For this review, take the finished solid that the model builds, in its own axes (mm). A direction names the side the tool comes from. Round coordinates to 2 decimals unless told otherwise and drop trailing zeros. Order: outer loops, then holes, each group sorted by start corner. A loop starts at its lowest first (then second) coordinate and runs counter-clockwise, first axis right, second up. Notation, with made-up numbers: (80.5, 82) - (103.5, 82) arc R27 ccw to (103.5, 109) - close; hole circle Ø7 at (72.5, 80.25). An arc over 180 degrees is marked (long way). One line per question, with ' | ' between items.
```python
from build123d import *

# Parameters (mm, degrees)
SKETCH1_R           = 23
SKETCH1_R_2         = 21
BOSS_EXTRUDE1_DEPTH = 20
CUT_EXTRUDE1_START  = 19.798989767
CUT_EXTRUDE1_DEPTH  = 3.113888708
BOSS_EXTRUDE2_START = -1
SKETCH3_R           = 21
SKETCH3_R_2         = 6
BOSS_EXTRUDE2_DEPTH = 1
BOSS_EXTRUDE3_START = 8
SKETCH4_R           = 6
BOSS_EXTRUDE3_DEPTH = 8


# Read off the part's stored shape, not the designer's step: Cut-Extrude1
with BuildPart() as part:
    # Sketch1 → Boss-Extrude1 (new body)
    with BuildSketch(Plane(origin=(0, 0, 0), x_dir=(0, 0, -1), z_dir=(1, 0, 0))):
        Circle(SKETCH1_R)
        Circle(SKETCH1_R_2, mode=Mode.SUBTRACT)
    extrude(amount=BOSS_EXTRUDE1_DEPTH)

    # Cut-Extrude1 outline → Cut-Extrude1 (cut)
    with BuildSketch(Plane(origin=(0, 0, 0), x_dir=(1, 0, 0), z_dir=(0, 1, 0)).offset(CUT_EXTRUDE1_START)):
        with BuildLine():
            add(Edge.make_bspline(
                [(7.15, 7), (7.818022917, 7), (8.466048034, 6.72160004), (9.377693338, 5.805707302), (9.644739555, 5.166655745), (9.655100007, 3.873398622), (9.398895769, 3.221423625), (8.466344312, 2.273000364), (7.817770221, 2), (7.15, 2)],
                knots=[0, 0, 0, 0, 0.25, 0.25, 0.5, 0.5, 0.75, 0.75, 1, 1, 1, 1], degree=3))
            Line((7.15, 7), (3.85, 7))
            add(Edge.make_bspline(
                [(3.85, 7), (3.181977083, 7), (2.533951966, 6.72160004), (1.622306662, 5.805707302), (1.355260445, 5.166655745), (1.344899993, 3.873398622), (1.601104231, 3.221423625), (2.533655688, 2.273000364), (3.182229779, 2), (3.85, 2)],
                knots=[0, 0, 0, 0, 0.25, 0.25, 0.5, 0.5, 0.75, 0.75, 1, 1, 1, 1], degree=3))
            Line((3.85, 2), (7.15, 2))
        make_face()
        with BuildLine():
            Line((3.85, -7), (7.15, -7))
            add(Edge.make_bspline(
                [(7.15, -7), (7.818022917, -7), (8.466048034, -6.72160004), (9.377693338, -5.805707302), (9.644739555, -5.166655745), (9.655100007, -3.873398622), (9.398895769, -3.221423625), (8.466344312, -2.273000364), (7.817770221, -2), (7.15, -2)],
                knots=[0, 0, 0, 0, 0.25, 0.25, 0.5, 0.5, 0.75, 0.75, 1, 1, 1, 1], degree=3))
            Line((7.15, -2), (3.85, -2))
            add(Edge.make_bspline(
                [(3.85, -7), (3.181977083, -7), (2.533951966, -6.72160004), (1.622306662, -5.805707302), (1.355260445, -5.166655745), (1.344899993, -3.873398622), (1.601104231, -3.221423625), (2.533655688, -2.273000364), (3.182229779, -2), (3.85, -2)],
                knots=[0, 0, 0, 0, 0.25, 0.25, 0.5, 0.5, 0.75, 0.75, 1, 1, 1, 1], degree=3))
        make_face()
    extrude(amount=CUT_EXTRUDE1_DEPTH, mode=Mode.SUBTRACT)

    # Sketch3 → Boss-Extrude2 (add)
    with BuildSketch(Plane(origin=(20, 0, 0), x_dir=(0, 0, -1), z_dir=(1, 0, 0)).offset(BOSS_EXTRUDE2_START)):
        Circle(SKETCH3_R)
        Circle(SKETCH3_R_2, mode=Mode.SUBTRACT)
    extrude(amount=BOSS_EXTRUDE2_DEPTH)

    # Sketch4 → Boss-Extrude3 (add)
    with BuildSketch(Plane.ZY.offset(-19).offset(BOSS_EXTRUDE3_START)):
        with BuildLine():
            Line((7.937253933, -1), (20.976176963, -1))
            ThreePointArc((20.976176963, -1), (21, 0), (20.976176963, 1))
            Line((20.976176963, 1), (7.937253933, 1))
            ThreePointArc((7.937253933, 1), (5.656854249, 5.656854249), (1, 7.937253933))
            Line((1, 7.937253933), (1, 20.976176963))
            ThreePointArc((1, 20.976176963), (0, 21), (-1, 20.976176963))
            Line((-1, 20.976176963), (-1, 7.937253933))
            ThreePointArc((-1, 7.937253933), (-5.656854249, 5.656854249), (-7.937253933, 1))
            Line((-7.937253933, 1), (-20.976176963, 1))
            ThreePointArc((-20.976176963, 1), (-21, 0), (-20.976176963, -1))
            Line((-20.976176963, -1), (-7.937253933, -1))
            ThreePointArc((-7.937253933, -1), (-5.656854249, -5.656854249), (-1, -7.937253933))
            Line((-1, -7.937253933), (-1, -20.976176963))
            ThreePointArc((-1, -20.976176963), (0, -21), (1, -20.976176963))
            Line((1, -20.976176963), (1, -7.937253933))
            ThreePointArc((1, -7.937253933), (5.656854249, -5.656854249), (7.937253933, -1))
        make_face()
        with Locations(Location((0, 0, 0), (0, 0, 180))):
            Circle(SKETCH4_R, mode=Mode.SUBTRACT)
    extrude(amount=-BOSS_EXTRUDE3_DEPTH)


solid = part.part
```
(1) Insertion check: pin 1 (3 mm diameter, centred on x = 10, y = 8, fed in from +Z); pin 2 (2.5 mm diameter, centred on x = 13.5, z = 15.5, fed in from +Y); pin 3 (10 mm diameter, centred on x = 7, y = -16, fed in from +Z). Each pin has a flat end and moves straight along its axis. Give the tip position at first contact, or say it passes through.
Output values:
pin 1: z = 22.06 | pin 2: y = 18.05 | pin 3: z = 20.2
(2) We need section D-D on x = 13.5. State the section outline as (y, z) points, plus the area to 3 significant figures.
Output values:
outline: circle Ø46 at (0, 0); hole (-20.98, -1) arc R21 ccw to (-1, -20.98) - (-1, -7.94) arc R8 cw to (-7.94, -1) - close; hole (-20.98, 1) - (-7.94, 1) arc R8 cw to (-1, 7.94) - (-1, 20.98) arc R21 ccw to start; hole circle Ø12 at (0, 0); hole (1, -20.98) arc R21 ccw to (20.98, -1) - (7.94, -1) arc R8 cw to (1, -7.94) - close; hole (1, 7.94) arc R8 cw to (7.94, 1) - (20.98, 1) arc R21 ccw to (1, 20.98) - close | area: 469 mm^2
(3) Mouldability with a two-part tool opening along Y and no side actions: class faces 1 (the flat face through (6, 21, -7)), 2 (the flat face through (15, 1, 15)) as released by +Y, released by -Y, zero draft, split by the parting line, or undercut.
Output values:
face 1: zero draft | face 2: undercut
(4) We need section C-C on x = 4.75. State the section outline as (y, z) points, plus the area to 3 significant figures.
Output values:
outline: (19.8, -7) arc R21 cw (long way) to (19.8, 7) - (21.91, 7) arc R23 ccw (long way) to (21.91, -7) - close; (20.9, -2) - (22.91, -2) arc R23 ccw to (22.91, 2) - (20.9, 2) arc R21 cw to start | area: 256 mm^2
(5) We need section A-A on z = 0. State the section outline as (x, y) points, plus the area to 3 significant figures.
Output values:
outline: (0, -23) - (20, -23) - (20, -6) - (11, -6) - (11, -21) - (0, -21) - close; (0, 21) - (11, 21) - (11, 6) - (20, 6) - (20, 23) - (0, 23) - close | area: 350 mm^2
(6) For faces 3 (the flat face through (19, -11, 11)), 4 (the flat face through (6, 22, 2)), 5 (the flat face through (0, -19, -10)), list the 3-axis set-ups (+Z, -Z, +X, -X, +Y, -Y) from which the entire face can be reached by the end or side of a thin tool; tool diameter is ignored.
Output values:
face 3: -X | face 4: +Y | face 5: +Z, -Z, -X, +Y, -Y
(7) For probe 1 along Z at (x, y) = (16, -10); probe 2 along Y at (x, z) = (19.45, 0); probe 3 along Y at (x, z) = (7.25, 0), list the stretches that pass through material, from the lowest coordinate up. Write a range as [from, to].
Output values:
probe 1: [-20.71, -18.47], [-1, 1], [18.47, 20.71] | probe 2: [-23, -6], [6, 23] | probe 3: [-23, -21], [21, 23]
